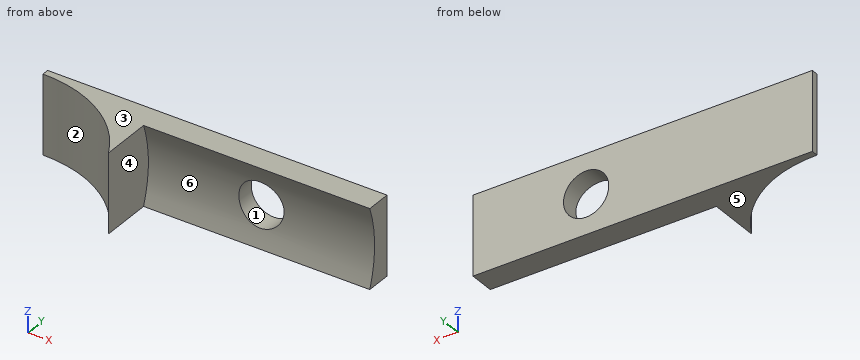
```python
from build123d import *

# Parameters (mm, degrees)
CYLINDER001_R          = 11.2
CYLINDER001_DEPTH      = 7
CYLINDER002_R          = 2
CYLINDER002_DEPTH      = 10
CYLINDER002_ROLL_ANGLE = -90
CYLINDER_R             = 10.2
CYLINDER_DEPTH         = 20
CYLINDER_PITCH_ANGLE   = 90
BOX_W                  = 30
BOX_H                  = 11.8
BOX_DEPTH              = 7


with BuildPart() as cylinder001:
    # Cylinder001 → Cylinder001 (new body)
    with BuildSketch(Plane.XY.offset(-3.5)):
        Circle(CYLINDER001_R)
    extrude(amount=CYLINDER001_DEPTH)


with BuildPart() as cylinder002:
    # Cylinder002 → Cylinder002 (new body)
    with BuildSketch(Plane.XY):
        Circle(CYLINDER002_R)
    extrude(amount=CYLINDER002_DEPTH)


with BuildPart() as cylinder002_1:
    # Cylinder002 roll: moved
    add(cylinder002.part.rotate(Axis((0, 0, 0), (1, 0, 0)), CYLINDER002_ROLL_ANGLE))


with BuildPart() as cylinder002_2:
    # Cylinder002 placement: moved
    add(cylinder002_1.part.moved(Location((20, 5, 0))))


with BuildPart() as fusion:
    # Cylinder → Cylinder (new body)
    with BuildSketch(Plane.XY):
        Circle(CYLINDER_R)
    extrude(amount=CYLINDER_DEPTH)


with BuildPart() as fusion_1:
    # Cylinder pitch: moved
    add(fusion.part.rotate(Axis((0, 0, 0), (0, 1, 0)), CYLINDER_PITCH_ANGLE))


with BuildPart() as fusion_2:
    # Cylinder placement: moved
    add(fusion_1.part.moved(Location((10, 0, 0))))

    # Fusion: union Cylinder001, Cylinder002
    add(cylinder001.part)
    add(cylinder002_2.part)


with BuildPart() as cut:
    # Box → Box (new body)
    with BuildSketch(Plane.XY.offset(-3.5)):
        with Locations((15, 5.9)):
            Rectangle(BOX_W, BOX_H)
    extrude(amount=BOX_DEPTH)

    # Cut: cut Fusion
    add(fusion_2.part, mode=Mode.SUBTRACT)


solid = cut.part
```
Can you work these out from the model? Positions are in its coordinate system, mm. Face numbers are marked on the shaded views. A direction names the side the tool comes from. Give positions to 0.01 mm unless a question says otherwise; leave off trailing zeros. Write each loop counter-clockwise with the first axis right and the second up, starting at its lowest first coordinate (ties: lowest second). Pieces come first, ordered by that corner, then holes. Notation, with made-up numbers: (20.5, 64.5) -> (74.5, 64.5) arc R30 cw to (74.5, 88.5) -> close; hole circle Ø9 at (-37.75, -5). An arc over 180 degrees is marked (long way). Write item = value, one per line.
(1) Suppose I cut it at A-A on x = 20. Write out the boundary of the cut face in (y, z), then the cut area to 3 significant figures.
Worked out:
outline = (9.58, -3.5) -> (11.8, -3.5) -> (11.8, -2) -> (10, -2) arc R10.2 cw to start; (9.58, 3.5) arc R10.2 cw to (10, 2) -> (11.8, 2) -> (11.8, 3.5) -> close
area = 5.96 mm^2
(2) Suppose I cut it at C-C on y = 10.75. Write out the boundary of the cut face in (x, z).
Worked out:
outline = (3.14, -3.5) -> (30, -3.5) -> (30, 3.5) -> (3.14, 3.5) -> close; hole circle Ø4 at (20, 0)
(3) Thinking about a two-plate mould opening in X: for the marked faces 1, 2, 3 and 4, which applies, released by +X, released by -X, zero draft, split by the parting line, or undercut?
Worked out:
face_1 = undercut
face_2 = released by -X
face_3 = zero draft
face_4 = released by +X
(4) Suppose I cut it at D-D on x = 24.5. Write out the boundary of the cut face in (y, z).
Worked out:
outline = (9.58, -3.5) -> (11.8, -3.5) -> (11.8, 3.5) -> (9.58, 3.5) arc R10.2 cw to start
(5) I need wall thicknesses on probe 1 along Z at (x, y) = (20, 11.1); probe 2 along X at (y, z) = (10, 0); probe 3 along Y at (x, z) = (17, -0.25). Which ranges of each line are inside material? Lowest first, please. Write a range as from..to.
Worked out:
probe_1 = -3.5..-2, 2..3.5
probe_2 = 5.04..10
probe_3 = 10.2..11.8
(6) For the marked faces 5 and 6, which set-ups out of +Z, -Z, +X, -X, +Y, -Y let a thin tool reach every point of the face, with its end or its side?
Worked out:
face_5 = -Z, +X, -X, +Y, -Y
face_6 = +X, -Y
(7) Suppose I cut it at B-B on z = 0. Write out the boundary of the cut face in (x, y).
Worked out:
outline = (0, 11.2) arc R11.2 cw to (10, 5.04) -> (10, 10.2) -> (18, 10.2) -> (18, 11.8) -> (0, 11.8) -> close; (22, 10.2) -> (30, 10.2) -> (30, 11.8) -> (22, 11.8) -> close
(8) I'm going to push a flat-ended pin straight in: P1, Ø1, axis at y = 7, z = -1.5, coming from the +X side. Where does the tip first touch, or does it pass through?
Worked out:
P1 = 10
